Read the model definition and answer for the solid it produces. Units are mm, in the model's axes. A direction names the side the tool comes from. Coordinates: 2 decimals unless noted, no trailing zeros. Order: outer loops, then holes, each group sorted by start corner. A loop starts at its lowest first (then second) coordinate and runs counter-clockwise, first axis right, second up.
Autodesk Inventor part; units mm, degrees
ref_plane "YZ Plane" through (0, 0, 0) normal (1, 0, 0) x (0, 1, 0)
ref_plane "XZ Plane" through (0, 0, 0) normal (0, 1, 0) x (-1, 0, 0)
ref_plane "XY Plane" through (0, 0, 0) normal (0, 0, 1) x (1, 0, 0)
sketch "Szkic1" plane through (0, 0, 0) normal (0, 0, 1) x (1, 0, 0)
  circle A0 centre (0, 0) radius 2.5
  line L0 (-2, 6.95) -> (2, 6.95)
  line L1 (-2, -6.95) -> (2, -6.95)
  line L2 (-2, 6.95) -> (-2, 5.6569)
  line L3 (2, 6.95) -> (2, 5.6569)
  line L4 (-2, -6.95) -> (-2, -5.6569)
  line L5 (2, -6.95) -> (2, -5.6569)
  arc A1 (-2, 5.6569) -> (-2, -5.6569) centre (0, 0) ccw
  arc A2 (2, -5.6569) -> (2, 5.6569) centre (0, 0) ccw
  circle A3 centre (2.55, 3.6469) radius 0.55
  circle A4 centre (4.2238, 1.4007) radius 0.55
  circle A5 centre (4.2238, -1.4006) radius 0.55
  circle A6 centre (2.55, -3.6469) radius 0.55
  circle A7 centre (-2.55, 3.6469) radius 0.55
  circle A8 centre (-4.2238, 1.4007) radius 0.55
  circle A9 centre (-4.2238, -1.4006) radius 0.55
  circle A10 centre (-2.55, -3.6469) radius 0.55
  dimension "d4" = 4
  dimension "d5" = 4
  dimension "d25" = 110.076
extrude "Wyciągnięcie proste3" add sketch "Szkic1" against normal blind 0.5
sketch "Szkic3" plane through (0, 0, -0.5) normal (0, 0, -1) x (-1, 0, 0)
  line L0 (2, 6.95) -> (-2, 6.95)
  line L1 (-2, 6.95) -> (2, 6.95)
  line L2 (2, 6.95) -> (2, 6.45)
  line L3 (2, 6.45) -> (-2, 6.45)
  line L4 (-2, 6.45) -> (-2, 6.95)
  line L5 (-2, -6.95) -> (2, -6.95)
  line L6 (-2, -6.95) -> (2, -6.95)
  line L7 (2, -6.95) -> (2, -6.45)
  line L8 (2, -6.45) -> (-2, -6.45)
  line L9 (-2, -6.45) -> (-2, -6.95)
extrude "Wyciągnięcie proste4" add sketch "Szkic3" along normal blind 0.75
fillet "Zaokrąglenie3" radius 0.25 4 edges at (-2, 5.6569, -0.25) (2, 5.6569, -0.25) (2, -5.6569, -0.25) (-2, -5.6569, -0.25)
fillet "Zaokrąglenie4" radius 0.5 2 edges at (0, -6.95, 0) (0, 6.95, 0)
properties part number "SŁONECZKO MAŁE" material "Stal"
1) Straight lines are drawn through the part: line 1 (Y direction, x = 3, z = -0.25); line 2 (Y direction, x = -0.75, z = -0.55); line 3 (Y direction, x = 2.55, z = -0.2). For each, find the intervals that lie inside material, in ascending order.
A:
line 1: y = -5.2 to -3.96, -3.33 to 3.33, 3.96 to 5.2
line 2: y = -6.95 to -6.45, 6.45 to 6.95
line 3: y = -5.43 to -4.2, -3.1 to 3.1, 4.2 to 5.43
2) A cutting plane is placed at D-D, the plane x = -1.25. Determine the outline of the cut face in (y, z), and give its area (3 significant figures).
A:
outline: (-6.95, -1.25) - (-6.45, -1.25) - (-6.45, -0.5) - (-2.17, -0.5) - (-2.17, 0) - (-6.45, 0) arc R0.5 ccw to (-6.95, -0.5) - close; (2.17, -0.5) - (6.45, -0.5) - (6.45, -1.25) - (6.95, -1.25) - (6.95, -0.5) arc R0.5 ccw to (6.45, 0) - (2.17, 0) - close
area: 5.43 mm2
3) A cutting plane is placed at C-C, the plane y = 0. Determine the outline of the cut face in (x, z).
A:
outline: (-6, -0.5) - (-2.5, -0.5) - (-2.5, 0) - (-6, 0) - close; (2.5, -0.5) - (6, -0.5) - (6, 0) - (2.5, 0) - close
4) Flat-ended cylindrical pins translate along their axes: pin 1 Ø0.6 at (y, z) = (-6.5, -1) entering from -X; pin 2 Ø1.8 at (x, y) = (2.55, 3.65) entering from -Z; pin 3 Ø0.6 at (y, z) = (-6.5, -1) entering from +X. Find the tip coordinate at first contact, or state that the pin passes through.
A:
pin 1: stops at x = -2
pin 2: stops at z = -0.5
pin 3: stops at x = 2
5) A cutting plane is placed at A-A, the plane x = 0. Determine the outline of the cut face in (y, z).
A:
outline: (-6.95, -1.25) - (-6.45, -1.25) - (-6.45, -0.5) - (-2.5, -0.5) - (-2.5, 0) - (-6.45, 0) arc R0.5 ccw to (-6.95, -0.5) - close; (2.5, -0.5) - (6.45, -0.5) - (6.45, -1.25) - (6.95, -1.25) - (6.95, -0.5) arc R0.5 ccw to (6.45, 0) - (2.5, 0) - close
6) Determine the mould class of faces 1 (the cylindrical face through (6, -0.1, -0.2)), 2 (the flat face through (-2, -6.65, -0.48)), 3 (the cylindrical face through (-4.6, 1.8, -0.2)) for opening direction Y: pulls with the +Y half, pulls with the -Y half, needs draft (parallel to the pull), parting line crosses it, or undercut.
A:
face 1: parting line crosses it
face 2: needs draft
face 3: undercut
7) Which of the six approach directions +Z, -Z, +X, -X, +Y, -Y give full straight-line access (tool end or side, diameter ignored) to faces 4 (the flat face through (-2, 6.65, -0.48)), 5 (the flat face through (2, -6.65, -0.48)), 6 (the flat face through (2, 6.65, -0.48))?
A:
face 4: +Z, -Z, -X, +Y
face 5: +Z, -Z, +X, -Y
face 6: +Z, -Z, +X, +Y
8) A cutting plane is placed at B-B, the plane z = -0.9. Determine the outline of the cut face in (x, y).
A:
outline: (-2, -6.95) - (2, -6.95) - (2, -6.45) - (-2, -6.45) - close; (-2, 6.45) - (2, 6.45) - (2, 6.95) - (-2, 6.95) - close
